from build123d import *

# Parameters (mm, degrees)
SKETCH007_R             = 2.75
PAD004_DEPTH            = 8
POCKET003_DEPTH         = 3
SKETCH013_R             = 4
SKETCH013_R_2           = 2.75
PAD009_DEPTH            = 1
SKETCH014_R             = 3.5
SKETCH014_R_2           = 2.75
PAD010_DEPTH            = 0.3
SKETCH015_R             = 4
SKETCH015_R_2           = 2.75
PAD011_DEPTH            = 8
SKETCH016_R             = 3.5
SKETCH016_R_2           = 2.75
PAD012_DEPTH            = 0.4
SKETCH018_R             = 6
POCKET005_DEPTH         = 2
POCKET006_DEPTH         = 3
SKETCH022_W             = 7
SKETCH022_H             = 20
PAD015_DEPTH            = 8
BODY001_ROLL_ANGLE      = 180
BODY001_PLACEMENT_ANGLE = -90


with BuildPart() as part:
    # Sketch007 → Pad004 (new body)
    with BuildSketch(Plane.XY):
        Polygon((0, 27.5), (43.9, 27.5), (56.4, 15), (56.4, 0), (0, 0), align=None)
        with Locations((16, 22)):
            Circle(SKETCH007_R, mode=Mode.SUBTRACT)
        with Locations((16, 10)):
            Circle(SKETCH007_R, mode=Mode.SUBTRACT)
        with Locations((38, 23.5)):
            Circle(SKETCH007_R, mode=Mode.SUBTRACT)
        with Locations((32.7, 7)):
            Circle(SKETCH007_R, mode=Mode.SUBTRACT)
        with Locations((50.95, 10.55)):
            Circle(SKETCH007_R, mode=Mode.SUBTRACT)
    extrude(amount=PAD004_DEPTH)

    # Sketch012 (on Face11 of Pad004) → Pocket003 (cut)
    with BuildSketch(Plane(origin=(0, 0, 0), x_dir=(1, 0, 0), z_dir=(0, 0, -1))):
        with BuildLine():
            ThreePointArc((40.45, -10.55), (43.525379, -17.974621), (50.95, -21.05))
            Line((50.95, -21.05), (70.95, -21.05))
            Line((70.95, -21.05), (70.95, 0))
            Line((70.95, 0), (40.45, 0))
            Line((40.45, -10.55), (40.45, 0))
        make_face()
    extrude(amount=-POCKET003_DEPTH, mode=Mode.SUBTRACT)

    # Sketch013 (on Face8 of Pocket003) → Pad009 (join)
    with BuildSketch(Plane(origin=(0, 0, 3), x_dir=(1, 0, 0), z_dir=(0, 0, -1))):
        with Locations((50.95, -10.55)):
            Circle(SKETCH013_R)
        with Locations((50.95, -10.55)):
            Circle(SKETCH013_R_2, mode=Mode.SUBTRACT)
    extrude(amount=PAD009_DEPTH)

    # Sketch014 (on Face16 of Pad009) → Pad010 (join)
    with BuildSketch(Plane(origin=(0, 0, 2), x_dir=(1, 0, 0), z_dir=(0, 0, -1))):
        with Locations((50.95, -10.55)):
            Circle(SKETCH014_R)
        with Locations((50.95, -10.55)):
            Circle(SKETCH014_R_2, mode=Mode.SUBTRACT)
    extrude(amount=PAD010_DEPTH)

    # Sketch015 (on Face4 of Pad010) → Pad011 (join)
    with BuildSketch(Plane(origin=(0, 0, 0), x_dir=(1, 0, 0), z_dir=(0, 0, -1))):
        with Locations((38, -23.5)):
            Circle(SKETCH015_R)
        with Locations((38, -23.5)):
            Circle(SKETCH015_R_2, mode=Mode.SUBTRACT)
    extrude(amount=PAD011_DEPTH)

    # Sketch016 (on Face17 of Pad011) → Pad012 (join)
    with BuildSketch(Plane(origin=(0, 0, -8), x_dir=(1, 0, 0), z_dir=(0, 0, -1))):
        with Locations((38, -23.5)):
            Circle(SKETCH016_R)
        with Locations((38, -23.5)):
            Circle(SKETCH016_R_2, mode=Mode.SUBTRACT)
    extrude(amount=PAD012_DEPTH)

    # Sketch018 (on Face5 of Pad012) → Pocket005 (cut)
    with BuildSketch(Plane.XY.offset(8)):
        with Locations((16, 10)):
            Circle(SKETCH018_R)
    extrude(amount=-POCKET005_DEPTH, mode=Mode.SUBTRACT)

    # Sketch019 (on Face5 of Pocket005) → Pocket006 (cut)
    with BuildSketch(Plane.XY.offset(8)):
        Polygon((20.75, 22), (18.375, 26.113621), (13.625, 26.113621), (11.25, 22), (13.625, 17.886379), (18.375, 17.886379), align=None)
        Polygon((42.75, 23.5), (40.375, 27.613621), (35.625, 27.613621), (33.25, 23.5), (35.625, 19.386379), (40.375, 19.386379), align=None)
        Polygon((37.45, 7), (35.075, 11.113621), (30.325, 11.113621), (27.95, 7), (30.325, 2.886379), (35.075, 2.886379), align=None)
        Polygon((55.7, 10.55), (53.325, 14.663621), (48.575, 14.663621), (46.2, 10.55), (48.575, 6.436379), (53.325, 6.436379), align=None)
    extrude(amount=-POCKET006_DEPTH, mode=Mode.SUBTRACT)

    # Sketch022 (on Face9 of Pocket006) → Pad015 (join)
    with BuildSketch(Plane.XZ):
        with Locations((29.7, -2)):
            Rectangle(SKETCH022_W, SKETCH022_H)
    extrude(amount=PAD015_DEPTH)


with BuildPart() as part_1:
    # Body001 roll: moved
    add(part.part.rotate(Axis((0, 0, 0), (1, 0, 0)), BODY001_ROLL_ANGLE))


with BuildPart() as part_2:
    # Body001 placement: moved
    add(part_1.part.moved(Location((65, 23, -20))).rotate(Axis((65, 23, -20), (0, 0, 1)), BODY001_PLACEMENT_ANGLE))


solid = part_2.part
Geometry: final body of the model. Coordinates: model frame, mm. A direction names the side the tool comes from. Give positions to 0.01 mm unless a question says otherwise; leave off trailing zeros. Write each loop counter-clockwise with the first axis right and the second up, starting at its lowest first coordinate (ties: lowest second). Pieces come first, ordered by that corner, then holes. Notation, with made-up numbers: (15, 42.25) -> (38, 42.25) arc R26 ccw to (38, 65.25) -> close; hole circle Ø1 at (6, 77.5). An arc over 180 degrees is marked (long way). Answer in a Markdown table with one row per item.
(1) Draft query along X for faces 4 (the cylindrical face through (41.676, -11.004, -16.056)), 5 (the flat face through (60.03, -6.12, -26.52)), 6 (the flat face through (53, -25, -21.7)). Return one class per face: +X half, -X half, draft (parallel to the pull), parting line (faces both ways), or undercut.
Answers below:
| item | result |
|---|---|
| face 4 | parting line |
| face 5 | undercut |
| face 6 | draft |
(2) Section query B-B on y = -27.95. Return loops of the section in (x, z), then the cut area to 3 significant figures.
Answers below:
| item | result |
|---|---|
| outline | (44.55, -28) -> (50.34, -28) -> (50.34, -25) -> (51.7, -25) -> (51.7, -21.7) -> (50.95, -21.7) -> (50.95, -22) -> (50.45, -22) -> (50.45, -23) -> (44.55, -23) -> close; (57.2, -25) -> (58.56, -25) -> (58.56, -28) -> (65, -28) -> (65, -23) -> (58.45, -23) -> (58.45, -22) -> (57.95, -22) -> (57.95, -21.7) -> (57.2, -21.7) -> close |
| area | 69.5 mm^2 |
(3) Set-up query: faces 1 (the flat face through (40.97, 3.42, -26.52)), 2 (the flat face through (43.7, -27.1, -24.8)), 3 (the flat face through (69, -3.2, -18)). Return all of +Z, -Z, +X, -X, +Y, -Y with unobstructed straight access to the full face (end or side cutting, diameter ignored); none if empty.
Answers below:
| item | result |
|---|---|
| face 1 | -Z |
| face 2 | +Z, -Z, -X, -Y |
| face 3 | +Z, -Z, +X, +Y |
(4) Pin query (flat end, axial travel): pin 1 (6.5 mm diameter, centred on y = 13, z = -22.5, fed in from +X); pin 2 (1 mm diameter, centred on y = -16, z = -15, fed in from +X); pin 3 (9 mm diameter, centred on x = 69.5, z = -16, fed in from -Y). Return the tip coordinate at first contact, or that it passes through.
Answers below:
| item | result |
|---|---|
| pin 1 | x = 65 |
| pin 2 | x = 45.47 |
| pin 3 | y = -10.2 |
(5) Section query A-A on z = -18. Return loops of the section in (x, y), then the cut area to 3 significant figures.
Answers below:
| item | result |
|---|---|
| outline | circle Ø8 at (41.5, -15); (65, -10.2) -> (73, -10.2) -> (73, -3.2) -> (65, -3.2) -> close; hole circle Ø5.5 at (41.5, -15) |
| area | 82.5 mm^2 |
(6) Ray query, line 1 along X through (y, z) = (-9.7, -22.75); line 2 along Y through (x, z) = (43, -21.7); line 3 along Y through (x, z) = (41.5, -18.25). Return the intervals inside material, ascending. Write a range as [from, to].
Answers below:
| item | result |
|---|---|
| line 1 | [37.5, 55.25], [60.75, 73] |
| line 2 | [-26.4, -17.3], [-12.7, 4.25], [9.75, 23] |
| line 3 | [-19, -17.75], [-12.25, -11] |
(7) Section query C-C on y = -4. Return loops of the section in (x, z).
Answers below:
| item | result |
|---|---|
| outline | (37.5, -28) -> (73, -28) -> (73, -8) -> (65, -8) -> (65, -20) -> (37.5, -20) -> close |
(8) Section query D-D on x = 69.5. Return loops of the section in (y, z), then the cut area to 3 significant figures.
Answers below:
| item | result |
|---|---|
| outline | (-10.2, -28) -> (-3.2, -28) -> (-3.2, -8) -> (-10.2, -8) -> close |
| area | 140 mm^2 |
